Part model, mm, in its own coordinate system. A direction names the side the tool comes from. Round coordinates to 2 decimals unless told otherwise and drop trailing zeros. Write each loop counter-clockwise with the first axis right and the second up, starting at its lowest first coordinate (ties: lowest second). Pieces come first, ordered by that corner, then holes.
Autodesk Inventor part; units mm, degrees
ref_plane "YZ Plane" through (0, 0, 0) normal (1, 0, 0) x (0, 1, 0)
ref_plane "XZ Plane" through (0, 0, 0) normal (0, 1, 0) x (-1, 0, 0)
ref_plane "XY Plane" through (0, 0, 0) normal (0, 0, 1) x (1, 0, 0)
sketch "Sketch1" plane through (0, 0, 0) normal (0, 1, 0) x (-1, 0, 0)
  line L0 (-7.5, 6) -> (7.5, 6)
  line L1 (7.5, 6) -> (7.5, -6)
  line L2 (7.5, -6) -> (-7.5, -6)
  line L3 (-7.5, -6) -> (-7.5, 6)
  line L4 (-7.5, 6) -> (7.5, -6) construction
  line L5 (7.5, 6) -> (-7.5, -6) construction
  point P0 (0, 0)
  dimension "d0" = 12
  dimension "d1" = 15
extrude "Extrusion1" add sketch "Sketch1" along normal mid plane 5
sketch "Sketch2" plane through (0, 2.5, 0) normal (0, 1, 0) x (1, 0, 0)
  line L0 (-5, 6) -> (-7.5, 6)
  line L1 (-7.5, 6) -> (-7.5, -6)
  line L2 (-7.5, -6) -> (-5, -6)
  line L3 (-5, -6) -> (-5, 6)
  line L4 (-5, 6) -> (-7.5, -6) construction
  line L5 (-7.5, 6) -> (-5, -6) construction
  line L6 (7.5, -6) -> (7.5, 6)
  line L7 (5, 6) -> (7.5, 6)
  line L8 (7.5, 6) -> (7.5, -6)
  line L9 (7.5, -6) -> (5, -6)
  line L10 (5, -6) -> (5, 6)
  line L11 (5, 6) -> (7.5, -6) construction
  line L12 (7.5, 6) -> (5, -6) construction
  line L13 (5, 0) -> (-5, 0) construction
  point P0 (0, 0)
  point P1 (-6.25, 0)
  point P2 (6.25, 0)
  point P3 (0, 0)
  dimension "d15" = 10
extrude "Extrusion2" add sketch "Sketch2" along normal blind 3
sketch "Sketch3" plane through (0, -2.5, 0) normal (0, -1, 0) x (1, 0, 0)
  point P0 (0, 0)
hole "Hole1" at (0, -2.5, 0) direction (0, 1, 0) diameter 3.797 end through all
mirror "Mirror1" about plane through (0, 0, 0) normal (0, 1, 0)
sketch "Sketch4" plane through (-5, 2.5, 6) normal (0, 0, 1) x (1, 0, 0)
  line L0 (-2.5, 3) -> (-2.5, -8)
  line L1 (-10.5, -8) -> (-2.5, -8)
  line L2 (-2.5, -8) -> (-2.5, 3)
  line L3 (-2.5, 3) -> (-10.5, 3)
  line L4 (-10.5, 3) -> (-10.5, -8)
  line L5 (-10.5, -8) -> (-2.5, 3) construction
  line L6 (-2.5, -8) -> (-10.5, 3) construction
  line L7 (-2.5, -8) -> (0, -8)
  point P0 (5, -2.5)
  point P1 (-6.5, -2.5)
  dimension "d16" = 8
extrude "Extrusion3" add sketch "Sketch4" against normal blind 5
sketch "Sketch5" plane through (-5, 2.5, 1) normal (0, 0, -1) x (-1, 0, 0)
  line L0 (10.5, -8) -> (10.5, 3)
  line L1 (2.5, -8) -> (10.5, -8)
  circle A0 centre (6.5, -2.5) radius 2.55
  point P0 (-5, -2.5)
  point P1 (10.5, -2.5)
  point P2 (6.5, -8)
  point P3 (10.5, -2.5)
  point P4 (6.5, -8)
  point P5 (6.5, -8)
  dimension "d19" = 5.1
extrude "Extrusion4" cut sketch "Sketch5" against normal through all
fillet "Fillet1" radius 2 2 edges at (-15.5, 5.5, 3.5) (-15.5, -5.5, 3.5)
properties part number "StopRotation"
Q1. Drop flat-ended pins along their axis: P1, Ø3.5, axis at y = 4.5, z = -1, coming from the -X side; P2, Ø5, axis at x = 0, y = 4, coming from the -Z side; P3, Ø3, axis at x = 0, z = 1.5, coming from the -Y side. Give the stop position or say it passes through.
Q2. Two-plate mould, pull along X, no slides. Class faces 1 (the flat face through (-2.2, 2.5, 0.1)), 2 (the flat face through (5, -4, 0)), 3 (the flat face through (7.5, 0, 0)), 4 (the flat face through (6, 5.5, 0)): released by +X, released by -X, zero draft, split by the parting line, or undercut.
Q3. Wall check: line 1 (Y direction, x = -11.5, z = 4.95); line 2 (X direction, y = -3, z = 1.5); line 3 (Z direction, x = 0, y = -0.4). Give the ranges that are in metal, low to high.
Q4. Saw through at C-C, the plane z = 3.25. Write the cut outline in (x, y), and give its area (3 significant figures).
Q5. Saw through at D-D, the plane z = -2.75. Write the cut outline in (x, y), and give its area (3 significant figures).
Q6. Saw through at B-B, the plane x = 0. Write the cut outline in (y, z), and give its area (3 significant figures).
Q7. Saw through at A-A, the plane y = 0. Write the cut outline in (x, z).
Q8. Tool access for faces 5 (the flat face through (-2.2, -2.5, 0.1)), 6 (the flat face through (-11, 3, 1)), 7 (the flat face through (5, 4, 0)), 8 (the cylindrical face through (1.853, 0.035, 0.412)): list every direction of +Z, -Z, +X, -X, +Y, -Y with a clear straight run to the whole face (end or side of a thin tool).
Computed:
1. P1: stops at x = -7.5
1. P2: stops at z = -6
1. P3: stops at y = -2.5
2. face 1: undercut
2. face 2: undercut
2. face 3: released by +X
2. face 4: zero draft
3. line 1: y = -5.5 to -2.55, 2.55 to 5.5
3. line 2: x = -15.5 to -5, 5 to 7.5
3. line 3: z = -6 to -1.9, 1.9 to 6
4. outline: (-15.5, -3.5) arc R2 ccw to (-13.5, -5.5) - (-5, -5.5) - (-5, -2.5) - (5, -2.5) - (5, -5.5) - (7.5, -5.5) - (7.5, 5.5) - (5, 5.5) - (5, 2.5) - (-5, 2.5) - (-5, 5.5) - (-13.5, 5.5) arc R2 ccw to (-15.5, 3.5) - close; hole circle Ø5.1 at (-11.5, 0)
4. area: 171 mm2
5. outline: (-7.5, -5.5) - (-5, -5.5) - (-5, -2.5) - (5, -2.5) - (5, -5.5) - (7.5, -5.5) - (7.5, 5.5) - (5, 5.5) - (5, 2.5) - (-5, 2.5) - (-5, 5.5) - (-7.5, 5.5) - close
5. area: 105 mm2
6. outline: (-2.5, -6) - (2.5, -6) - (2.5, -1.9) - (-2.5, -1.9) - close; (-2.5, 1.9) - (2.5, 1.9) - (2.5, 6) - (-2.5, 6) - close
6. area: 41.0 mm2
7. outline: (-15.5, 1) - (-14.05, 1) - (-14.05, 6) - (-15.5, 6) - close; (-8.95, 1) - (-7.5, 1) - (-7.5, -6) - (7.5, -6) - (7.5, 6) - (-8.95, 6) - close; hole circle Ø3.8 at (0, 0)
8. face 5: +Z, -Z, -Y
8. face 6: -Z, -X, +Y, -Y
8. face 7: +Z, -Z, +Y
8. face 8: +Y, -Y
